For this review, use the dimensioned drawing (mm, ordinates from the lowest corner) and the shaded views. A direction names the side the tool comes from. Round coordinates to 2 decimals unless told otherwise and drop trailing zeros. Loops run counter-clockwise (first coordinate to the right, second up) from the corner with the lowest first, then second, coordinate; pieces in that order, holes last. Notation, with made-up numbers: M -27,37.5 L -10,37.5 A29 ccw -10,69.5 Z; hole C -33.5,-6 d8. An arc over 180 degrees is marked long. One line per item, written item: value. Start each with the question number.
Item 1: For the marked faces 5 and 6, list the 3-axis set-ups (+Z, -Z, +X, -X, +Y, -Y) from which the entire face can be reached by the end or side of a thin tool; tool diameter is ignored.
Item 2: Clearance check with flat-ended pins moving along their axes: pin 1 (2 mm diameter, centred on y = 31.5, z = 11, fed in from -X); pin 2 (2 mm diameter, centred on y = 6.5, z = 12.5, fed in from +X); pin 3 (12 mm diameter, centred on y = 31.5, z = 4, fed in from -X); pin 4 (4 mm diameter, centred on y = 11.5, z = 13.99, fed in from +X). State where each tip first meets the part, or that it passes through.
Item 3: We need section B-B (x = 4.25). Write out the cut boundary in (y, z).
Item 4: Mouldability with a two-part tool opening along Z and no side actions: class the marked faces 1, 2, 3 and 4 as released by +Z, released by -Z, zero draft, split by the parting line, or undercut.
Item 5: We need section A-A (z = 3). Write out the cut boundary in (x, y), then the cut area to 3 significant figures.
Item 6: For line 1 along X through (y, z) = (19.5, 22.25); line 2 along Y through (x, z) = (9, 13.5); line 3 along Y through (x, z) = (1.25, 13.75) (1 decimal), list the stretches that pass through material, from the lowest coordinate up.
Item 7: We need section D-D (x = 9.5). Write out the cut boundary in (y, z), then the cut area to 3 significant figures.
Item 8: We need section C-C (y = 7.5). Write out the cut boundary in (x, z), then the cut area to 3 significant figures.
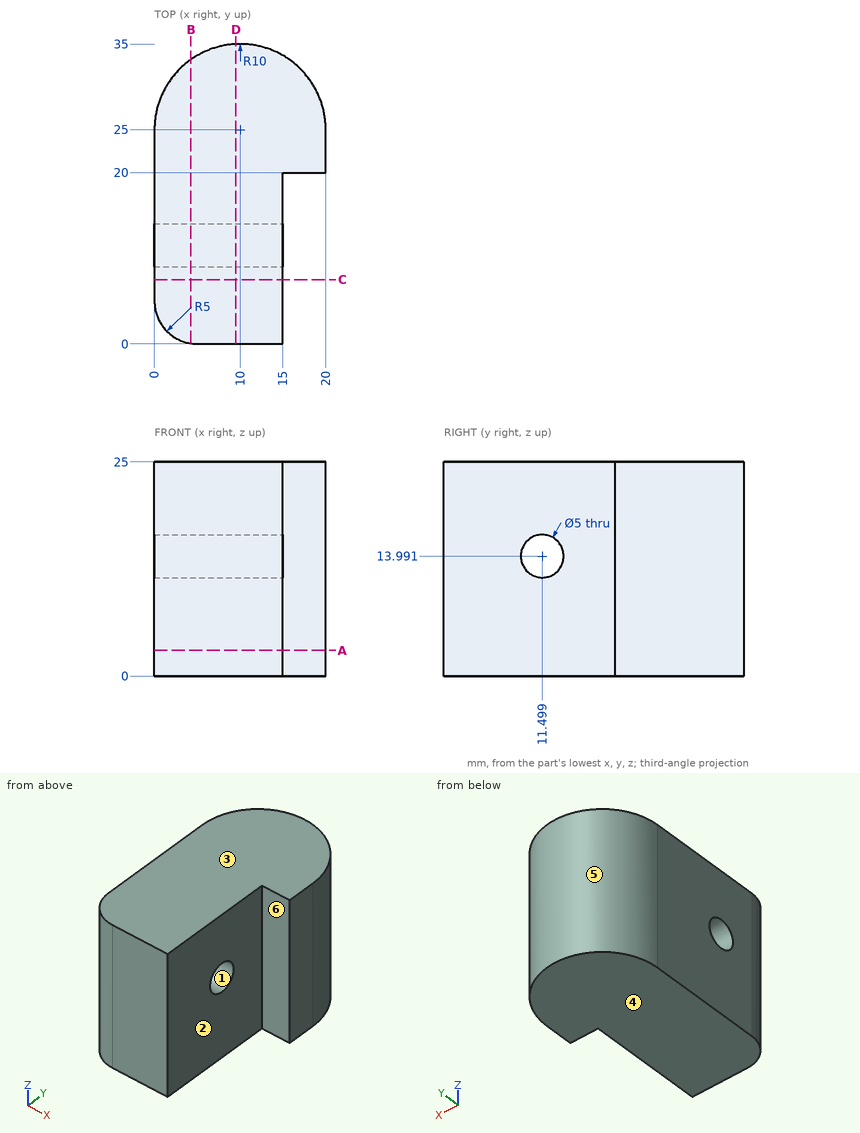
A:
1. face 5: +Z, -Z, +Y
1. face 6: +Z, -Z, +X, -Y
2. pin 1: x = 1.65
2. pin 2: x = 15
2. pin 3: x = 0.01
2. pin 4: through
3. outline: M 0.06,0 L 33.18,0 L 33.18,25 L 0.06,25 Z; hole C 11.5,13.99 d5
4. face 1: undercut
4. face 2: zero draft
4. face 3: released by +Z
4. face 4: released by -Z
5. outline: M 0,5 A5 ccw 5,0 L 15,0 L 15,20 L 20,20 L 20,25 A10 ccw 0,25 Z
5. area: 552 mm2
6. line 1: 0 to 15
6. line 2: 0 to 9.05, 13.95 to 34.95
6. line 3: 1.7 to 9, 14 to 29.8
7. outline: M 0,0 L 34.99,0 L 34.99,25 L 0,25 Z; hole C 11.5,13.99 d5
7. area: 855 mm2
8. outline: M 0,0 L 15,0 L 15,25 L 0,25 Z
8. area: 375 mm2
